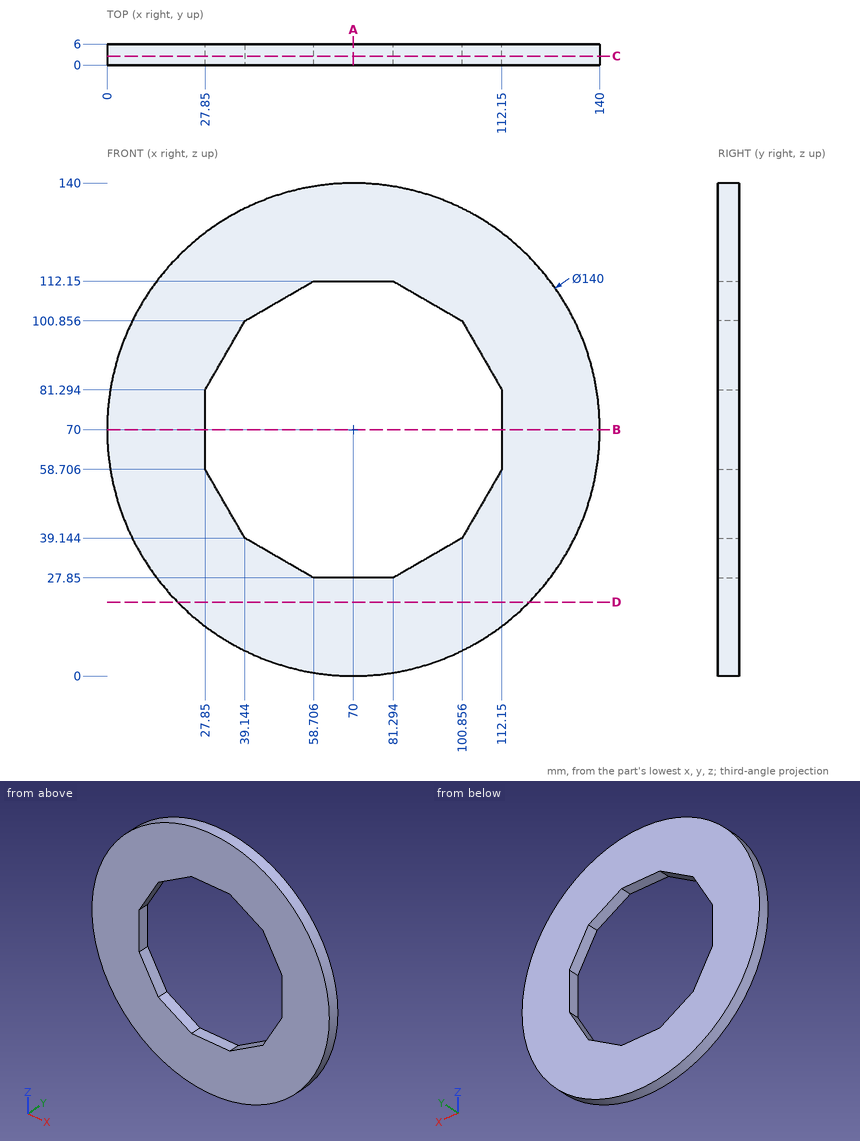
The drawing under review shows one solid part. Ordinate dimensions are in mm from its lowest x, y, z. Round coordinates to 2 decimals unless told otherwise and drop trailing zeros. Write each loop counter-clockwise with the first axis right and the second up, starting at its lowest first coordinate (ties: lowest second). Pieces come first, ordered by that corner, then holes. Notation, with made-up numbers: (36.25, 79.5) -> (88.25, 79.5) arc R29 ccw to (88.25, 105.5) -> close; hole circle Ø10 at (-12, 12.5). An arc over 180 degrees is marked (long way). One line per question, with ' | ' between items.
(1) Take a section at D-D, the plane z = 21. State the section outline as (x, y) points.
Result sheet:
outline: (20.01, 0) -> (119.99, 0) -> (119.99, 6) -> (20.01, 6) -> close
(2) Take a section at A-A, the plane x = 70. State the section outline as (y, z) points.
Result sheet:
outline: (0, 0) -> (6, 0) -> (6, 27.85) -> (0, 27.85) -> close; (0, 112.15) -> (6, 112.15) -> (6, 140) -> (0, 140) -> close
(3) Insertion check: P1, Ø4, axis at x = 114.5, z = 82, coming from the -Y side; P2, Ø1.8, axis at y = 4, z = 73.5, coming from the -X side; P3, Ø1.8, axis at y = 1.5, z = 67.5, coming from the +X side; P4, Ø1.5, axis at y = 5, z = 21, coming from the +X side. Each pin has a flat end and moves straight along its axis. Give the tip position at first contact, or say it passes through.
Result sheet:
P1: y = 0 | P2: x = 0.05 | P3: x = 139.98 | P4: x = 120.71
(4) Take a section at B-B, the plane z = 70. State the section outline as (x, y) points, and give its area (3 significant figures).
Result sheet:
outline: (0, 0) -> (27.85, 0) -> (27.85, 6) -> (0, 6) -> close; (112.15, 0) -> (140, 0) -> (140, 6) -> (112.15, 6) -> close | area: 334 mm2
(5) Wall thickness on line 1 (Z direction, x = 72, y = 4.6); line 2 (Z direction, x = 97, y = 5.5): over which ranges is each line inside the solid? List them lowest first. Write a range as [from, to].
Result sheet:
line 1: [0.03, 27.85], [112.15, 139.97] | line 2: [5.42, 36.92], [103.08, 134.58]
(6) Take a section at C-C, the plane y = 2.55. State the section outline as (x, z) points, and give its area (3 significant figures).
Result sheet:
outline: circle Ø140 at (70, 70); hole (27.85, 58.71) -> (39.14, 39.14) -> (58.71, 27.85) -> (81.29, 27.85) -> (100.86, 39.14) -> (112.15, 58.71) -> (112.15, 81.29) -> (100.86, 100.86) -> (81.29, 112.15) -> (58.71, 112.15) -> (39.14, 100.86) -> (27.85, 81.29) -> close | area: 9,680 mm2
